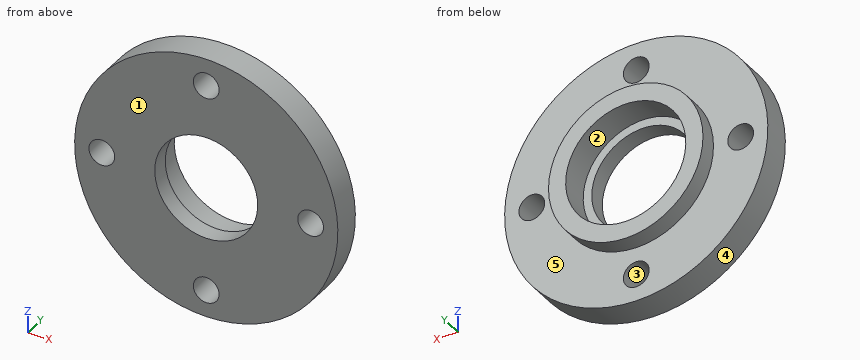
from build123d import *

# Parameters (mm, degrees)
M4_CLEARANCE_HOLE1_D = 4.5
CIRPATTERN1_COUNT    = 4


with BuildPart() as part:
    # Sketch1 → Revolve1 (revolve)
    with BuildSketch(Plane.XY, mode=Mode.PRIVATE) as revolve1_sk:
        Polygon((9, 0), (9, -3), (23, -3), (23, 2), (13.5, 2), (13.5, 5), (10.5, 5), (10.5, 0), align=None)
    revolve(revolve1_sk.sketch.rotate(Axis((0, -55, 0), (0, 1, 0)), 90), axis=Axis((0, -55, 0), (0, 1, 0)))

    # M4 Clearance Hole1 (through all)
    with Locations(Plane(origin=(0, 2, 0), x_dir=(1, 0, 0), z_dir=(0, 1, 0))):
        with Locations((18.25, 0)):
            m4_clearance_hole1 = Hole(M4_CLEARANCE_HOLE1_D / 2)

    # CirPattern1: M4 Clearance Hole1 ×4 about axis
    cirpattern1_axis = Axis((0, 0, 0), (0, 1, 0))
    for i in range(1, CIRPATTERN1_COUNT):
        add(m4_clearance_hole1.rotate(cirpattern1_axis, i * 360 / CIRPATTERN1_COUNT), mode=Mode.SUBTRACT)


solid = part.part
Model file for the job. Use its own axes, mm. Face numbers are marked on the shaded views. A direction names the side the tool comes from. Coordinates: 2 decimals unless noted, no trailing zeros. Write each loop counter-clockwise with the first axis right and the second up, starting at its lowest first coordinate (ties: lowest second). Pieces come first, ordered by that corner, then holes. Notation, with made-up numbers: (82.5, 6.5) -> (110.5, 6.5) arc R20 ccw to (110.5, 13.5) -> close; hole circle Ø5 at (-29, -40). An arc over 180 degrees is marked (long way). One line per item, written item: value. Start each with the question number.
1) Slice it at C-C on z = 5. Write the cut outline in (x, y).
2) Flat gauge pins, fed straight in: pin 1 Ø16 at (x, z) = (0, 0) entering from +Y; pin 2 Ø1 at (x, y) = (-17, -0.5) entering from -Z; pin 3 Ø6 at (x, z) = (0, 18.25) entering from +Y; pin 4 Ø3 at (x, y) = (-3.5, -2) entering from +Z. Where does each tip first touch, or does it go through?
3) Slice it at D-D on x = 18.25. Write the cut outline in (y, z).
4) Slice it at A-A on z = 0. Write the cut outline in (x, y), then the cut area to 3 significant figures.
5) Slice it at B-B on y = -2. Write the cut outline in (x, z), then the cut area to 3 significant figures.
6) Pull direction Z, two halves, no side cores. Call the marked faces 3, 4 and 5: +Z half, -Z half, draft (parallel to the pull), parting line (faces both ways), or undercut.
7) Probe probe 1 along X at (y, z) = (-2, -1.5); probe 2 along Y at (x, z) = (-4.5, -18); probe 3 along X at (y, z) = (-0.75, 3). List the from-to ranges inside material, lowest first.
8) Which spindle directions (+Z, -Z, +X, -X, +Y, -Y) get a long thin tool onto all of the face, cutting with end or side? Do the marked faces 1 and 2. Say none if no direction does.
Answers follow:
1. outline: (-22.45, -3) -> (-7.48, -3) -> (-7.48, 0) -> (-9.23, 0) -> (-9.23, 5) -> (-12.54, 5) -> (-12.54, 2) -> (-22.45, 2) -> close; (7.48, -3) -> (22.45, -3) -> (22.45, 2) -> (12.54, 2) -> (12.54, 5) -> (9.23, 5) -> (9.23, 0) -> (7.48, 0) -> close
2. pin 1: through
2. pin 2: z = -16.02
2. pin 3: y = 2
2. pin 4: z = 22.91
3. outline: (-3, -14) -> (2, -14) -> (2, -2.25) -> (-3, -2.25) -> close; (-3, 2.25) -> (2, 2.25) -> (2, 14) -> (-3, 14) -> close
4. outline: (-23, -3) -> (-20.5, -3) -> (-20.5, 2) -> (-23, 2) -> close; (-16, -3) -> (-9, -3) -> (-9, 0) -> (-10.5, 0) -> (-10.5, 5) -> (-13.5, 5) -> (-13.5, 2) -> (-16, 2) -> close; (9, -3) -> (16, -3) -> (16, 2) -> (13.5, 2) -> (13.5, 5) -> (10.5, 5) -> (10.5, 0) -> (9, 0) -> close; (20.5, -3) -> (23, -3) -> (23, 2) -> (20.5, 2) -> close
4. area: 107 mm2
5. outline: circle Ø46 at (0, 0); hole circle Ø4.5 at (-18.25, 0); hole circle Ø18 at (0, 0); hole circle Ø4.5 at (0, -18.25); hole circle Ø4.5 at (0, 18.25); hole circle Ø4.5 at (18.25, 0)
5. area: 1,340 mm2
6. face 3: undercut
6. face 4: parting line
6. face 5: draft
7. probe 1: -22.95 to -19.93, -16.57 to -8.87, 8.87 to 16.57, 19.93 to 22.95
7. probe 2: -3 to 2
7. probe 3: -22.8 to -8.49, 8.49 to 22.8
8. face 1: +Z, -Z, +X, -X, -Y
8. face 2: +Y
